Check sheet for the modelled part. Datum: model origin and axes. Units: mm. A direction names the side the tool comes from. Give positions to 0.01 mm unless a question says otherwise; leave off trailing zeros. Write each loop counter-clockwise with the first axis right and the second up, starting at its lowest first coordinate (ties: lowest second). Pieces come first, ordered by that corner, then holes. Notation, with made-up numbers: (38, 84.5) - (59, 84.5) arc R24 cw to (59, 102.5) - close; hole circle Ø7 at (40, -2). An arc over 180 degrees is marked (long way). Return JSON: item names as keys, results as strings. Group by question number.
```python
from build123d import *

# Parameters (mm, degrees)
SKETCH1_R           = 84
SKETCH1_R_2         = 79.22
SKETCH3_R           = 84
SKETCH3_R_2         = 79.22
BOSS_EXTRUDE1_DEPTH = 600
SKETCH4_R           = 127.5
SKETCH4_R_2         = 79.22
SKETCH4_R_3         = 6
BOSS_EXTRUDE2_DEPTH = 8


with BuildPart() as part:
    # Sweep1: sweep along a path in Sketch2
    with BuildLine(Plane.XY) as sweep1_path:
        ThreePointArc((0, 0), (66.955389821, 161.644610179), (228.6, 228.6))
    # Sketch1 → Sweep1 (sweep)
    with BuildSketch(Plane(origin=(0, 0, 0), x_dir=(1, 0, 0), z_dir=(0, 1, 0))):
        Circle(SKETCH1_R)
        Circle(SKETCH1_R_2, mode=Mode.SUBTRACT)
    sweep(path=sweep1_path.line)

    # Sketch3 → Boss-Extrude1 (add)
    with BuildSketch(Plane(origin=(228.6, 0, 0), x_dir=(0, 0, -1), z_dir=(1, 0, 0))):
        with Locations(Location((0, 228.6, 0), (0, 0, 90))):
            Circle(SKETCH3_R)
        with Locations(Location((0, 228.6, 0), (0, 0, 90))):
            Circle(SKETCH3_R_2, mode=Mode.SUBTRACT)
    extrude(amount=BOSS_EXTRUDE1_DEPTH)

    # Sketch4 → Boss-Extrude2 (add)
    with BuildSketch(Plane(origin=(828.6, 0, 0), x_dir=(0, 0, -1), z_dir=(1, 0, 0))):
        with Locations(Location((0, 228.6, 0), (0, 0, 90))):
            Circle(SKETCH4_R)
        with Locations(Location((0, 228.6, 0), (0, 0, 90))):
            Circle(SKETCH4_R_2, mode=Mode.SUBTRACT)
        with Locations(Location((0, 337.6, 0), (0, 0, 90))):
            Circle(SKETCH4_R_3, mode=Mode.SUBTRACT)
        with Locations(Location((77.074639149, 305.674639149, 0), (0, 0, 90))):
            Circle(SKETCH4_R_3, mode=Mode.SUBTRACT)
        with Locations(Location((109, 228.6, 0), (0, 0, 90))):
            Circle(SKETCH4_R_3, mode=Mode.SUBTRACT)
        with Locations(Location((77.074639149, 151.525360851, 0), (0, 0, 90))):
            Circle(SKETCH4_R_3, mode=Mode.SUBTRACT)
        with Locations(Location((0, 119.6, 0), (0, 0, 90))):
            Circle(SKETCH4_R_3, mode=Mode.SUBTRACT)
        with Locations(Location((-77.074639149, 151.525360851, 0), (0, 0, 90))):
            Circle(SKETCH4_R_3, mode=Mode.SUBTRACT)
        with Locations(Location((-109, 228.6, 0), (0, 0, 90))):
            Circle(SKETCH4_R_3, mode=Mode.SUBTRACT)
        with Locations(Location((-77.074639149, 305.674639149, 0), (0, 0, 90))):
            Circle(SKETCH4_R_3, mode=Mode.SUBTRACT)
    extrude(amount=BOSS_EXTRUDE2_DEPTH)


solid = part.part
```
Item 1: Depth check by flat-ended pin: pin 1 (19 mm diameter, centred on y = 151.53, z = -77.07, fed in from +X); pin 2 (2 mm diameter, centred on x = 84, z = -65, fed in from +Y); pin 3 (14 mm diameter, centred on y = 119.6, z = 0, fed in from -X); pin 4 (3 mm diameter, centred on x = 366.5, y = 265.5, fed in from -Z). Enter the tip coordinate at first touch or a pass-through.
Item 2: Mould release check, pull along X, two halves, no side actions. Record for faces 1 (the face through (836.6, 170, -55)), 2 (the face through (832.54, 346.38, -48.83)), 3 (the face through (828.6, 142, 2)): +X half, -X half, draft (parallel to the pull), parting line (faces both ways), or undercut.
Item 3: Section check B-B on x = 313.5. Record the cut outline in (y, z), plus the area to 3 significant figures.
Item 4: Section check A-A on z = 20. Record the cut outline in (x, y), plus the area to 3 significant figures.
Item 5: Material ranges on line 1 along Z through (x, y) = (835, 228.6); line 2 along Z through (x, y) = (665, 228); line 3 along X through (y, z) = (128.5, -31.5), recorded low to high. Write a range as from..to.
Item 6: Access from +Z, -Z, +X, -X, +Y, -Y to the whole of each face (thin tool, end or side, straight path). Record for faces 4 (the face through (62, 0, -50)), 5 (the face through (528.344, 149.457, 3.483)), 6 (the face through (524.4, 144.68, 3.69)).
Reply:
{
 "1": {"pin 1": "x = 836.6", "pin 2": "y = 243.4", "pin 3": "x = -63.02", "pin 4": "z = -76.18"},
 "2": {"face 1": "+X half", "face 2": "draft", "face 3": "undercut"},
 "3": {"outline": "circle Ø168 at (228.6, 0); hole circle Ø158.44 at (228.6, 0)", "area": "2,450 mm²"},
 "4": {"outline": "(-81.58, 0) - (-76.65, 0) arc R305.25 cw to (228.6, 305.25) - (836.6, 305.25) - (836.6, 354.52) - (828.6, 354.52) - (828.6, 310.18) - (228.6, 310.18) arc R310.18 ccw to start; (76.65, 0) - (81.58, 0) arc R147.02 cw to (228.6, 147.02) - (828.6, 147.02) - (828.6, 102.68) - (836.6, 102.68) - (836.6, 151.95) - (228.6, 151.95) arc R151.95 ccw to start", "area": "10,200 mm²"},
 "5": {"line 1": "-127.5..-115, -103..-79.22, 79.22..103, 115..127.5", "line 2": "-84..-79.22, 79.22..84", "line 3": "-49.63..-43.91, 140.3..149.81, 828.6..836.6"},
 "6": {"face 4": "+Z, -Z, +X, -X, -Y", "face 5": "+X", "face 6": "none"}
}
